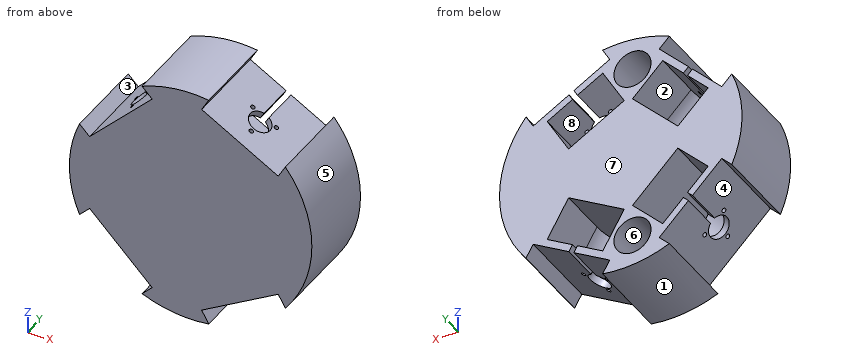
from build123d import *

# Parameters (mm, degrees)
BASE_DEPTH                = 60
MOTOR_TRASEIRO_START      = -5
MOTOR_TRASEIRO_DEPTH      = 30
ESBO_O3_10_R              = 1.5
MOTOR_EIXO_DEPTH          = 25
PADR_OCIRCULAR1_COUNT     = 2
PADR_OCIRCULAR1_ANGLE     = 285
ESPELHAR3_START           = -5
ESPELHAR3_COPY_1_DEPTH    = 30
ESPELHAR3_COPY_2_SKETCH_R = 1.5
ESPELHAR3_COPY_2_DEPTH    = 25
ESBO_O16_R                = 13
CAPACITORES_DEPTH         = 45


with BuildPart() as part:
    # Esboço1 → Base (new body)
    with BuildSketch(Plane(origin=(0, 0, 0), x_dir=(1, 0, 0), z_dir=(0, 1, 0))):
        with BuildLine():
            Line((-70.813516723, -26.97289629), (-26.97289629, -70.813516723))
            Line((-26.97289629, -70.813516723), (-34.043964102, -77.884584535))
            ThreePointArc((-34.043964102, -77.884584535), (-11.094726339, -84.272813217), (12.725930358, -84.041957953))
            Line((12.725930358, -84.041957953), (7.725930358, -75.381703915))
            Line((7.725930358, -75.381703915), (61.419505392, -44.381703915))
            Line((61.419505392, -44.381703915), (66.419505392, -53.041957953))
            ThreePointArc((66.419505392, -53.041957953), (85, 0), (66.419505392, 53.041957953))
            Line((66.419505392, 53.041957953), (61.419505392, 44.381703915))
            Line((61.419505392, 44.381703915), (7.725930358, 75.381703915))
            Line((7.725930358, 75.381703915), (12.725930358, 84.041957953))
            ThreePointArc((12.725930358, 84.041957953), (-11.094726339, 84.272813217), (-34.043964102, 77.884584535))
            Line((-34.043964102, 77.884584535), (-26.97289629, 70.813516723))
            Line((-26.97289629, 70.813516723), (-70.813516723, 26.97289629))
            Line((-70.813516723, 26.97289629), (-77.884584535, 34.043964102))
            ThreePointArc((-77.884584535, 34.043964102), (-85, 0), (-77.884584535, -34.043964102))
            Line((-77.884584535, -34.043964102), (-70.813516723, -26.97289629))
        make_face()
    extrude(amount=BASE_DEPTH)

    # Esboço3 → Motor-traseiro (cut)
    with BuildSketch(Plane(origin=(-48.893206507, 0, 48.893206507), x_dir=(0.7071067811865515, 0, 0.7071067811865436), z_dir=(-0.7071067811865436, 0, 0.7071067811865515)).offset(MOTOR_TRASEIRO_START)):
        with BuildLine():
            ThreePointArc((-22.5, 25), (0, 2.5), (22.5, 25))
            Line((22.5, 25), (22.5, 80))
            Line((22.5, 80), (-22.5, 80))
            Line((-22.5, 80), (-22.5, 25))
        make_face()
    motor_traseiro = extrude(amount=-MOTOR_TRASEIRO_DEPTH, mode=Mode.SUBTRACT)

    # Esboço3<10> → Motor-eixo (cut)
    with BuildSketch(Plane(origin=(-48.893206507, 0, 48.893206507), x_dir=(0.7071067811865515, 0, 0.7071067811865436), z_dir=(-0.7071067811865436, 0, 0.7071067811865515))):
        with BuildLine():
            Line((2, 32.745966692), (2, 70))
            Line((2, 70), (-2, 70))
            Line((-2, 70), (-2, 32.745966692))
            ThreePointArc((-2, 32.745966692), (0, 17), (2, 32.745966692))
        make_face()
        with Locations((0, 14)):
            Circle(ESBO_O3_10_R)
        with Locations((-9.526279442, 30.5)):
            Circle(ESBO_O3_10_R)
        with Locations((9.526279442, 30.5)):
            Circle(ESBO_O3_10_R)
    motor_eixo = extrude(amount=-MOTOR_EIXO_DEPTH, mode=Mode.SUBTRACT)

    # PadrãoCircular1: Motor-traseiro, Motor-eixo ×2 about axis
    padr_ocircular1_axis = Axis((0, 60, 0), (0, -1, 0))
    add([motor_traseiro.rotate(padr_ocircular1_axis, i * PADR_OCIRCULAR1_ANGLE / (PADR_OCIRCULAR1_COUNT - 1)) for i in range(1, PADR_OCIRCULAR1_COUNT)], mode=Mode.SUBTRACT)
    add([motor_eixo.rotate(padr_ocircular1_axis, i * PADR_OCIRCULAR1_ANGLE / (PADR_OCIRCULAR1_COUNT - 1)) for i in range(1, PADR_OCIRCULAR1_COUNT)], mode=Mode.SUBTRACT)

    # Espelhar3: Motor-traseiro, Motor-eixo across plane
    add(motor_traseiro.mirror(Plane.XY), mode=Mode.SUBTRACT)
    add(motor_eixo.mirror(Plane.XY), mode=Mode.SUBTRACT)

    # Espelhar3 copy 1 sketch → Espelhar3 copy 1 (cut)
    with BuildSketch(Plane(origin=(34.572717875, 0, -59.881703915), x_dir=(0.8660254037844427, 0, 0.499999999999993), z_dir=(0.499999999999993, 0, -0.8660254037844427)).offset(ESPELHAR3_START)):
        with BuildLine():
            ThreePointArc((-22.5, -25), (0, -2.5), (22.5, -25))
            Line((22.5, -25), (22.5, -80))
            Line((22.5, -80), (-22.5, -80))
            Line((-22.5, -80), (-22.5, -25))
        make_face()
    extrude(amount=-ESPELHAR3_COPY_1_DEPTH, mode=Mode.SUBTRACT)

    # Espelhar3 copy 2 sketch → Espelhar3 copy 2 (cut)
    with BuildSketch(Plane(origin=(34.572717875, 0, -59.881703915), x_dir=(0.8660254037844427, 0, 0.499999999999993), z_dir=(0.499999999999993, 0, -0.8660254037844427))):
        with BuildLine():
            Line((2, -32.745966692), (2, -70))
            Line((2, -70), (-2, -70))
            Line((-2, -70), (-2, -32.745966692))
            ThreePointArc((-2, -32.745966692), (0, -17), (2, -32.745966692))
        make_face()
        with Locations((0, -14)):
            Circle(ESPELHAR3_COPY_2_SKETCH_R)
        with Locations((-9.526279442, -30.5)):
            Circle(ESPELHAR3_COPY_2_SKETCH_R)
        with Locations((9.526279442, -30.5)):
            Circle(ESPELHAR3_COPY_2_SKETCH_R)
    extrude(amount=-ESPELHAR3_COPY_2_DEPTH, mode=Mode.SUBTRACT)

    # Esboço16 → Capacitores (cut)
    with BuildSketch(Plane(origin=(0, 60, 0), x_dir=(1, 0, 0), z_dir=(0, 1, 0))):
        with Locations(Location((-8.22315011, -62.461026267, 0), (0, 0, 270))):
            Circle(ESBO_O16_R)
        with Locations(Location((-8.22315011, 62.461026267, 0), (0, 0, 270))):
            Circle(ESBO_O16_R)
    extrude(amount=-CAPACITORES_DEPTH, mode=Mode.SUBTRACT)


solid = part.part
For this review, take the finished solid that the model builds, in its own axes (mm). Face numbers are marked on the shaded views. A direction names the side the tool comes from. Round coordinates to 2 decimals unless told otherwise and drop trailing zeros. Loops run counter-clockwise (first coordinate to the right, second up) from the corner with the lowest first, then second, coordinate; pieces in that order, holes last. Notation, with made-up numbers: (46, -34) - (57, -34) arc R21 ccw to (57, -22) - close; hole circle Ø3 at (-4.75, -6.75). An arc over 180 degrees is marked (long way). Put each result on its own line as item: value. Start each with the question number.
1. Consider section B-B on x = 55.5. State the section outline as (y, z) points, plus the area to 3 significant figures.
2. Mouldability with a two-part tool opening along Z and no side actions: class the marked faces 5, 6, 7 and 8 as +Z half, -Z half, draft (parallel to the pull), parting line (faces both ways), or undercut.
3. Insertion check: P1, Ø3, axis at x = 5, y = 6.5, coming from the -Z side; P2, Ø10, axis at x = -35, y = 33, coming from the -Z side; P3, Ø1.5, axis at x = 44, y = 53.5, coming from the -Z side. Each pin has a flat end and moves straight along its axis. Give the tip position at first contact, or say it passes through.
4. Consider section A-A on y = 51.5. State how many separate pieces and enclosed holes the cut face has, plus the area to 3 significant figures.
5. For the marked faces 1, 2, 3 and 4, list the 3-axis set-ups (+Z, -Z, +X, -X, +Y, -Y) from which the entire face can be reached by the end or side of a thin tool; tool diameter is ignored.
6. For probe 1 along X at (y, z) = (38.5, -19); probe 2 along Z at (x, y) = (6.5, 47); probe 3 along Z at (x, y) = (12, 41), list the stretches that pass through material, from the lowest coordinate up. Write a range as [from, to].
Result sheet:
1. outline: (0, -47.8) - (60, -47.8) - (60, 47.8) - (0, 47.8) - close
1. area: 5,740 mm^2
2. face 5: parting line
2. face 6: undercut
2. face 7: draft
2. face 8: undercut
3. P1: z = -84.93
3. P2: z = -79.53
3. P3: z = -54.87
4. separate pieces: 1
4. enclosed holes: 2
4. area: 12,700 mm^2
5. face 1: -Z, +Y, -Y
5. face 2: +Y
5. face 3: +Z, +Y, -Y
5. face 4: +Y, -Y
6. probe 1: [-82.85, -50.82], [-29.29, 35.38], [36.95, 82.85]
6. probe 2: [-84.75, -56.26], [-35.67, 35.67], [56.26, 84.75]
6. probe 3: [-84.15, -82.78], [-72.91, -65.78], [-32.5, 32.5], [65.78, 72.91], [82.78, 84.15]
